Check sheet for the modelled part. Datum: model origin and axes. Units: mm. A direction names the side the tool comes from. Coordinates: 2 decimals unless noted, no trailing zeros. Loops run counter-clockwise (first coordinate to the right, second up) from the corner with the lowest first, then second, coordinate; pieces in that order, holes last. Notation, with made-up numbers: M -11.75,74.25 L 10.25,74.25 A30 ccw 10.25,102.25 Z; hole C 16,76.5 d10. An arc over 180 degrees is marked long. Answer as CSV lines item,"result". Start each with the question number.
from build123d import *

# Parameters (mm, degrees)
F1_DEPTH = 5
F2_DEPTH = 3.5
F3_R     = 2
F4_R     = 23
F5_DEPTH = 5


# Not quite as in the source:
# - a feature names something its author has since deleted; it is built from what else it names


with BuildPart() as f1:
    # F0 (on Top) → F1 (new body)
    with BuildSketch(Plane.XY):
        with BuildLine():
            ThreePointArc((-25, 0), (-24.5524423049, 4.7093074719), (-23.2257938508, 9.25))
            Line((-23.2257938508, 9.25), (-34.5, 9.25))
            Line((-34.5, 9.25), (-34.5, -9.25))
            Line((-34.5, -9.25), (-23.2257938508, -9.25))
            ThreePointArc((-23.2257938508, -9.25), (-24.5524423049, -4.7093074719), (-25, 0))
        make_face()
        Polygon((-25, 6.25), (-25, 0), (-25, -6.25), (-31.5, -6.25), (-31.5, 6.25), align=None, mode=Mode.SUBTRACT)
        with BuildLine():
            Line((34.5, 9.25), (23.2257938508, 9.25))
            ThreePointArc((23.2257938508, 9.25), (24.5524423049, 4.7093074719), (25, 0))
            ThreePointArc((25, 0), (24.5524423049, -4.7093074719), (23.2257938508, -9.25))
            Line((23.2257938508, -9.25), (34.5, -9.25))
            Line((34.5, -9.25), (34.5, 9.25))
        make_face()
        Polygon((25, -6.25), (25, 0), (25, 6.25), (31.5, 6.25), (31.5, -6.25), align=None, mode=Mode.SUBTRACT)
        Polygon((-25, -6.25), (-25, 0), (-25, 6.25), (-31.5, 6.25), (-31.5, -6.25), align=None)
        Polygon((25, 6.25), (25, 0), (25, -6.25), (31.5, -6.25), (31.5, 6.25), align=None)
        with BuildLine():
            ThreePointArc((21.0579557412, 9.25), (22.5092534533, 4.7258342095), (23, 0))
            ThreePointArc((23, 0), (22.5092534533, -4.7258342095), (21.0579557412, -9.25))
            Line((21.0579557412, -9.25), (23.2257938508, -9.25))
            ThreePointArc((23.2257938508, -9.25), (24.5524423049, -4.7093074719), (25, 0))
            ThreePointArc((25, 0), (24.5524423049, 4.7093074719), (23.2257938508, 9.25))
            Line((23.2257938508, 9.25), (21.0579557412, 9.25))
        make_face()
        with BuildLine():
            ThreePointArc((9.25, 21.0579557412), (16.2634559673, 16.2634559673), (21.0579557412, 9.25))
            Line((21.0579557412, 9.25), (23.2257938508, 9.25))
            ThreePointArc((23.2257938508, 9.25), (17.6776695297, 17.6776695297), (9.25, 23.2257938508))
            Line((9.25, 23.2257938508), (9.25, 21.0579557412))
        make_face()
        with BuildLine():
            ThreePointArc((-21.0579557412, 9.25), (-16.2634559673, 16.2634559673), (-9.25, 21.0579557412))
            Line((-9.25, 21.0579557412), (-9.25, 23.2257938508))
            ThreePointArc((-9.25, 23.2257938508), (-17.6776695297, 17.6776695297), (-23.2257938508, 9.25))
            Line((-23.2257938508, 9.25), (-21.0579557412, 9.25))
        make_face()
        with BuildLine():
            Line((-9.25, -23.2257938508), (-9.25, -21.0579557412))
            ThreePointArc((-9.25, -21.0579557412), (-16.2634559673, -16.2634559673), (-21.0579557412, -9.25))
            Line((-21.0579557412, -9.25), (-23.2257938508, -9.25))
            ThreePointArc((-23.2257938508, -9.25), (-17.6776695297, -17.6776695297), (-9.25, -23.2257938508))
        make_face()
        with BuildLine():
            ThreePointArc((-21.0579557412, -9.25), (-23, 0), (-21.0579557412, 9.25))
            Line((-21.0579557412, 9.25), (-23.2257938508, 9.25))
            ThreePointArc((-23.2257938508, 9.25), (-24.5524423049, 4.7093074719), (-25, 0))
            ThreePointArc((-25, 0), (-24.5524423049, -4.7093074719), (-23.2257938508, -9.25))
            Line((-23.2257938508, -9.25), (-21.0579557412, -9.25))
        make_face()
        with BuildLine():
            ThreePointArc((-9.25, 21.0579557412), (0, 23), (9.25, 21.0579557412))
            Line((9.25, 21.0579557412), (9.25, 23.2257938508))
            ThreePointArc((9.25, 23.2257938508), (4.7093074719, 24.5524423049), (0, 25))
            ThreePointArc((0, 25), (-4.7093074719, 24.5524423049), (-9.25, 23.2257938508))
            Line((-9.25, 23.2257938508), (-9.25, 21.0579557412))
        make_face()
        with BuildLine():
            Line((23.2257938508, -9.25), (21.0579557412, -9.25))
            ThreePointArc((21.0579557412, -9.25), (16.2634559673, -16.2634559673), (9.25, -21.0579557412))
            Line((9.25, -21.0579557412), (9.25, -23.2257938508))
            ThreePointArc((9.25, -23.2257938508), (17.6776695297, -17.6776695297), (23.2257938508, -9.25))
        make_face()
        with BuildLine():
            Line((9.25, -23.2257938508), (9.25, -21.0579557412))
            ThreePointArc((9.25, -21.0579557412), (0, -23), (-9.25, -21.0579557412))
            Line((-9.25, -21.0579557412), (-9.25, -23.2257938508))
            ThreePointArc((-9.25, -23.2257938508), (-4.7093074719, -24.5524423049), (0, -25))
            ThreePointArc((0, -25), (4.7093074719, -24.5524423049), (9.25, -23.2257938508))
        make_face()
        with BuildLine():
            Line((9.25, -34.5), (9.25, -23.2257938508))
            ThreePointArc((9.25, -23.2257938508), (4.7093074719, -24.5524423049), (0, -25))
            ThreePointArc((0, -25), (-4.7093074719, -24.5524423049), (-9.25, -23.2257938508))
            Line((-9.25, -23.2257938508), (-9.25, -34.5))
            Line((-9.25, -34.5), (9.25, -34.5))
        make_face()
        Polygon((-6.25, -25), (0, -25), (6.25, -25), (6.25, -31.5), (-6.25, -31.5), align=None, mode=Mode.SUBTRACT)
        Polygon((6.25, -25), (0, -25), (-6.25, -25), (-6.25, -31.5), (6.25, -31.5), align=None)
        with BuildLine():
            ThreePointArc((0, 25), (4.7093074719, 24.5524423049), (9.25, 23.2257938508))
            Line((9.25, 23.2257938508), (9.25, 34.5))
            Line((9.25, 34.5), (-9.25, 34.5))
            Line((-9.25, 34.5), (-9.25, 23.2257938508))
            ThreePointArc((-9.25, 23.2257938508), (-4.7093074719, 24.5524423049), (0, 25))
        make_face()
        Polygon((6.25, 25), (0, 25), (-6.25, 25), (-6.25, 31.5), (6.25, 31.5), align=None, mode=Mode.SUBTRACT)
        Polygon((-6.25, 25), (0, 25), (6.25, 25), (6.25, 31.5), (-6.25, 31.5), align=None)
    extrude(amount=-F1_DEPTH)

    # F0 (on Top) → F2 (cut)
    with BuildSketch(Plane.XY):
        Polygon((-25, -6.25), (-25, 0), (-25, 6.25), (-31.5, 6.25), (-31.5, -6.25), align=None)
        Polygon((25, 6.25), (25, 0), (25, -6.25), (31.5, -6.25), (31.5, 6.25), align=None)
        Polygon((-6.25, 25), (0, 25), (6.25, 25), (6.25, 31.5), (-6.25, 31.5), align=None)
        Polygon((6.25, -25), (0, -25), (-6.25, -25), (-6.25, -31.5), (6.25, -31.5), align=None)
    extrude(amount=-F2_DEPTH, mode=Mode.SUBTRACT)

    # F3
    f3_edges = [f1.edges().sort_by_distance(p)[0] for p in [
        (-34.5, 9.25, -2.5),
        (-34.5, -9.25, -2.5),
        (34.5, 9.25, -2.5),
        (23.225794, -9.25, -2.5),
        (34.5, -9.25, -2.5),
        (-23.225794, -9.25, -2.5),
        (23.225794, 9.25, -2.5),
        (9.25, 34.5, -2.5),
        (9.25, 23.225794, -2.5),
        (9.25, -34.5, -2.5),
        (-9.25, -34.5, -2.5),
        (-9.25, -23.225794, -2.5),
        (9.25, -23.225794, -2.5),
        (-9.25, 34.5, -2.5),
        (-9.25, 23.225794, -2.5),
        (-23.225794, 9.25, -2.5),
    ]]
    fillet(f3_edges, radius=F3_R)

    # F4 (on face) → F5 (join)
    with BuildSketch(Plane(origin=(0, 0, -5), x_dir=(1, 0, 0), z_dir=(0, 0, -1))):
        with BuildLine():
            ThreePointArc((22.7264835722, -10.4166666667), (24.4250085906, -5.330943195), (25, 0))
            ThreePointArc((25, 0), (24.4250085906, 5.330943195), (22.7264835722, 10.4166666667))
            ThreePointArc((22.7264835722, 10.4166666667), (17.6776695297, 17.6776695297), (10.4166666667, 22.7264835722))
            ThreePointArc((10.4166666667, 22.7264835722), (0, 25), (-10.4166666667, 22.7264835722))
            ThreePointArc((-10.4166666667, 22.7264835722), (-17.6776695297, 17.6776695297), (-22.7264835722, 10.4166666667))
            ThreePointArc((-22.7264835722, 10.4166666667), (-25, 0), (-22.7264835722, -10.4166666667))
            ThreePointArc((-22.7264835722, -10.4166666667), (-17.6776695297, -17.6776695297), (-10.4166666667, -22.7264835722))
            ThreePointArc((-10.4166666667, -22.7264835722), (0, -25), (10.4166666667, -22.7264835722))
            ThreePointArc((10.4166666667, -22.7264835722), (17.6776695297, -17.6776695297), (22.7264835722, -10.4166666667))
        make_face()
        Circle(F4_R, mode=Mode.SUBTRACT)
    extrude(amount=F5_DEPTH)


solid = f1.part
Item 1: Go/stop test with flat-tipped pins: pin 1 (4 mm diameter, centred on x = -27.5, z = -1, fed in from +Y); pin 2 (2 mm diameter, centred on x = 27.5, y = -2.5, fed in from +Z); pin 3 (4 mm diameter, centred on y = 27, z = -2.5, fed in from +X). Record where each tip stops, or that it passes through.
Item 2: Sectioned sample at C-C, the plane z = -8.5. Record the boundary of the cut face in (x, y), and give its area (3 significant figures).
Item 3: Sectioned sample at A-A, the plane x = 0. Record the boundary of the cut face in (y, z), and give its area (3 significant figures).
Item 4: Sectioned sample at D-D, the plane z = -1. Give the number of separate pieces and of enclosed holes in the cut face, and give its area (3 significant figures).
Item 5: Sectioned sample at B-B, the plane y = -5. Record the boundary of the cut face in (x, z).
Item 6: Material ranges on line 1 (X direction, y = 27, z = -1.5); line 2 (X direction, y = 0, z = -8.8); line 3 (Z direction, x = 9, y = -23.5), recorded low to high. Write a range as from..to.
Item 7: Set-up check for faces 5 (the face through (33.9, -8.68, -2.54)), 6 (the face through (25, 0, -2)), 7 (the face through (9.25, 28, -2)), 8 (the face through (-28, 9.25, -2)): record each of +Z, -Z, +X, -X, +Y, -Y from which the full face is reachable in a straight line by a thin tool's end or side.
Item 8: Release check for a two-part mould opening along Y. For faces 1 (the face through (0, 34.5, -2)), 2 (the face through (-9.25, 29, -2)), 3 (the face through (0, 31.5, -2)), 4 (the face through (9.558, -23.478, -2.535)) record: released by +Y, released by -Y, zero draft, split by the parting line, or undercut.
Reply:
1,pin 1,"y = 9.25"
1,pin 2,"z = -3.5"
1,pin 3,"x = 9.25"
2,outline,"C 0,0 d50; hole C 0,0 d46"
2,area,"302 mm²"
3,outline,"M -34.5,-5 L -25,-5 L -25,-10 L -23,-10 L -23,0 L -25,0 L -25,-3.5 L -31.5,-3.5 L -31.5,0 L -34.5,0 Z; M 23,-10 L 25,-10 L 25,-5 L 34.5,-5 L 34.5,0 L 31.5,0 L 31.5,-3.5 L 25,-3.5 L 25,0 L 23,0 Z"
3,area,"89.5 mm²"
4,separate pieces,"1"
4,enclosed holes,"5"
4,area,"718 mm²"
5,outline,"M -34.5,-5 L -24.49,-5 L -24.49,-10 L -22.45,-10 L -22.45,0 L -25,0 L -25,-3.5 L -31.5,-3.5 L -31.5,0 L -34.5,0 Z; M 22.45,-10 L 24.49,-10 L 24.49,-5 L 34.5,-5 L 34.5,0 L 31.5,0 L 31.5,-3.5 L 25,-3.5 L 25,0 L 22.45,0 Z"
6,line 1,"-9.25..-6.25, 6.25..9.25"
6,line 2,"-25..-23, 23..25"
6,line 3,"-5..0"
7,face 5,"+Z, -Z, +X, -Y"
7,face 6,"+Z"
7,face 7,"+Z, -Z, +X, +Y"
7,face 8,"+Z, -Z, -X, +Y"
8,face 1,"released by +Y"
8,face 2,"zero draft"
8,face 3,"undercut"
8,face 4,"released by -Y"
